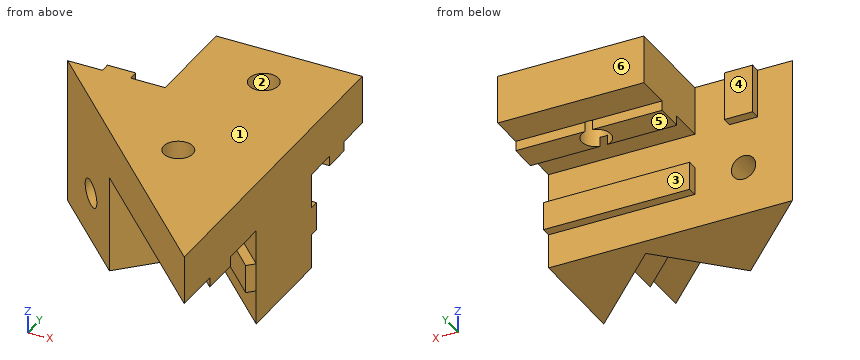
from build123d import *

# Parameters (mm, degrees)
MAIN_DEPTH          = 15
SKETCH4_W           = 15
SKETCH4_H           = 10
CUT_EXTRUDE2_DEPTH  = 10
SKETCH2_W           = 15
SKETCH2_H           = 2.9
BOSS_EXTRUDE3_DEPTH = 1
SKETCH5_W           = 2.9
SKETCH5_H           = 12.715728752
BOSS_EXTRUDE4_DEPTH = 1
SKETCH6_R           = 1.5
BOSS_EXTRUDE5_DEPTH = 5
BOSS_EXTRUDE6_DEPTH = 1
SKETCH8_W           = 2.9
SKETCH8_H           = 10
BOSS_EXTRUDE7_DEPTH = 1
SKETCH9_W           = 1
SKETCH9_H           = 2.9
BOSS_EXTRUDE8_DEPTH = 10
SKETCH11_R          = 1.25
CUT_EXTRUDE4_DEPTH  = 26
SKETCH12_R          = 1.5
CUT_EXTRUDE5_DEPTH  = 16
SKETCH13_W          = 15
SKETCH13_H          = 2.9
BOSS_EXTRUDE9_DEPTH = 1
SKETCH15_W          = 10
SKETCH15_H          = 10
CUT_EXTRUDE7_DEPTH  = 11
SKETCH16_R          = 1.5
CUT_EXTRUDE8_DEPTH  = 16
SKETCH14_W          = 30.791050847
SKETCH14_H          = 42.890305085
CUT_EXTRUDE6_DEPTH  = 26


with BuildPart() as part:
    # Sketch1 → Main (new body)
    with BuildSketch(Plane.XY):
        Polygon((0, 0), (-10, 0), (-10, 10), (-25, 10), (-25, -10.857864376), (-16.008621971, -1.866486348), (-8.937554159, -8.937554159), align=None)
    extrude(amount=MAIN_DEPTH)

    # Sketch4 → Cut-Extrude2 (cut)
    with BuildSketch(Plane(origin=(0, 0, 0), x_dir=(-1, 0, 0), z_dir=(0, 0, -1))):
        with Locations((17.5, 5)):
            Rectangle(SKETCH4_W, SKETCH4_H)
    extrude(amount=-CUT_EXTRUDE2_DEPTH, mode=Mode.SUBTRACT)

    # Sketch2 → Boss-Extrude3 (add)
    with BuildSketch(Plane(origin=(0, 0, 10), x_dir=(-1, 0, 0), z_dir=(0, 0, -1))):
        with Locations((17.5, 5)):
            Rectangle(SKETCH2_W, SKETCH2_H)
    extrude(amount=BOSS_EXTRUDE3_DEPTH)

    # Sketch5 → Boss-Extrude4 (add)
    with BuildSketch(Plane(origin=(-7.071067812, 7.071067812, 0), x_dir=(0, 0, -1), z_dir=(0.707106781, -0.707106781, 0))):
        with Locations((-5, -18.997474683)):
            Rectangle(SKETCH5_W, SKETCH5_H)
    extrude(amount=BOSS_EXTRUDE4_DEPTH)

    # Sketch6 → Boss-Extrude5 (add)
    with BuildSketch(Plane.XY.offset(10)):
        Polygon((-25, -10.857864376), (-16.008621971, -1.866486348), (-8.937554159, -8.937554159), (-25, -25), align=None)
        with Locations((-16.008621971, -8.937554159)):
            Circle(SKETCH6_R, mode=Mode.SUBTRACT)
    extrude(amount=BOSS_EXTRUDE5_DEPTH)

    # Sketch7 → Boss-Extrude6 (add)
    with BuildSketch(Plane(origin=(0, 0, 10), x_dir=(-1, 0, 0), z_dir=(0, 0, -1))):
        Polygon((13.498392898, -4.376715421), (25, -15.878322523), (25, -19.979541854), (11.447783233, -6.427325086), align=None)
    extrude(amount=BOSS_EXTRUDE6_DEPTH)

    # Sketch8 → Boss-Extrude7 (add)
    with BuildSketch(Plane(origin=(0, 0, 0), x_dir=(1, 0, 0), z_dir=(0, 1, 0))):
        with Locations((-5, -10)):
            Rectangle(SKETCH8_W, SKETCH8_H)
    extrude(amount=BOSS_EXTRUDE7_DEPTH)

    # Sketch11 → Cut-Extrude4 (cut, through all)
    with BuildSketch(Plane(origin=(0, 0, 0), x_dir=(1, 0, 0), z_dir=(0, 1, 0))):
        with Locations((-5, -5)):
            Circle(SKETCH11_R)
    extrude(amount=-CUT_EXTRUDE4_DEPTH, mode=Mode.SUBTRACT)

    # Sketch12 → Cut-Extrude5 (cut, through all)
    with BuildSketch(Plane.XY.offset(15)):
        with Locations((-16.008621971, -8.937554159)):
            Circle(SKETCH12_R)
    extrude(amount=-CUT_EXTRUDE5_DEPTH, mode=Mode.SUBTRACT)

    # Sketch13 → Boss-Extrude9 (add)
    with BuildSketch(Plane(origin=(0, 0, 0), x_dir=(1, 0, 0), z_dir=(0, 1, 0))):
        with Locations((-17.5, -5)):
            Rectangle(SKETCH13_W, SKETCH13_H)
    extrude(amount=BOSS_EXTRUDE9_DEPTH)


with BuildPart() as body_2:
    # Sketch9 → Boss-Extrude8 (new body)
    with BuildSketch(Plane.XY.offset(15)):
        with Locations((-9.5, 5)):
            Rectangle(SKETCH9_W, SKETCH9_H)
    extrude(amount=-BOSS_EXTRUDE8_DEPTH)


with BuildPart() as cut_extrude7_tool:
    # Sketch15 → Cut-Extrude7 (new body, through all)
    with BuildSketch(Plane(origin=(0, 0, 10), x_dir=(-1, 0, 0), z_dir=(0, 0, -1))):
        with Locations((5, 5)):
            Rectangle(SKETCH15_W, SKETCH15_H)
    extrude(amount=CUT_EXTRUDE7_DEPTH)


with BuildPart() as part_1:
    add(part.part)

    # Cut-Extrude7: cut by cut_extrude7_tool
    add(cut_extrude7_tool.part, mode=Mode.SUBTRACT)

    # Sketch16 → Cut-Extrude8 (cut, through all)
    with BuildSketch(Plane.XY.offset(15)):
        with Locations((-17.5, 5)):
            Circle(SKETCH16_R)
    extrude(amount=-CUT_EXTRUDE8_DEPTH, mode=Mode.SUBTRACT)


with BuildPart() as body_2_1:
    add(body_2.part)

    # Cut-Extrude7: cut by cut_extrude7_tool
    add(cut_extrude7_tool.part, mode=Mode.SUBTRACT)


with BuildPart() as body_3:
    # Mirror1: mirrored copy
    add(part_1.part.mirror(Plane.ZY.offset(30)))


with BuildPart() as cut_extrude6_tool:
    # Sketch14 → Cut-Extrude6 (new body, through all)
    with BuildSketch(Plane(origin=(-25, 0, -10), x_dir=(0, 0, -1), z_dir=(1, 0, 0))):
        with Locations((-11.471050848, -6.763186441)):
            Rectangle(SKETCH14_W, SKETCH14_H)
    extrude(amount=CUT_EXTRUDE6_DEPTH)


with BuildPart() as part_2:
    add(part_1.part)

    # Cut-Extrude6: cut by cut_extrude6_tool
    add(cut_extrude6_tool.part, mode=Mode.SUBTRACT)


with BuildPart() as body_2_2:
    add(body_2_1.part)

    # Cut-Extrude6: cut by cut_extrude6_tool
    add(cut_extrude6_tool.part, mode=Mode.SUBTRACT)


solid = body_3.part
Could you check a few things on this model? Use its own coordinates, in mm. Face numbers are marked on the shaded views. A direction names the side the tool comes from. Coordinates: 2 decimals unless noted, no trailing zeros. Order: outer loops, then holes, each group sorted by start corner. A loop starts at its lowest first (then second) coordinate and runs counter-clockwise, first axis right, second up. Notation, with made-up numbers: (63.5, -30.5) - (120.5, -30.5) arc R26 cw to (120.5, -9.5) - close; hole circle Ø2 at (53, -16.5). An arc over 180 degrees is marked (long way). Answer in a Markdown table with one row per item. Add a question column.
(1) If we mould it in two halves opening along Y, with no side actions, what happens to the marked faces 1, 2 and 3? For each: released by +Y, released by -Y, zero draft, split by the parting line, or undercut.
(2) If we section it at D-D, the plane z = 11: Please give me the cut outline in (x, y).
(3) Will these pins go through, and if not, where does the flat tip stop? pin 1 (0.8 mm diameter, centred on x = -46, z = 9.5, fed in from -Y); pin 2 (2 mm diameter, centred on x = -49.5, z = 7.5, fed in from -Y); pin 3 (10.5 mm diameter, centred on x = -42, y = -15.5, fed in from -Z); pin 4 (4 mm diameter, centred on x = -44.5, y = 1.5, fed in from -Z).
(4) If we section it at C-C, the plane z = 5: Please give me the cut outline in (x, y).
(5) On a 3-axis mill with a long thin cutter (end or side, diameter ignored), from which of +Z, -Z, +X, -X, +Y, -Y can I reach the whole of each face in a straight line? I mean the marked faces 4, 5 and 6. Say none if no direction works.
(6) I need wall thicknesses on L1, parallel to X at y = 5, z = 13.7; L2, parallel to X at y = -2.75, z = 5; L3, parallel to Z at x = -55, y = -1.25. Which ranges of each line are inside material? Lowest first, please.
(7) If we section it at B-B, the plane x = -54.25: Please give me the cut outline in (y, z), then the cut area to 4 significant figures.
(8) If we section it at A-A, the plane y = 5: Please give me the cut outline in (x, z), then the cut area to 3 significant figures.
Results are:
| question | item | result |
|---|---|---|
| 1 | face 1 | zero draft |
| 1 | face 2 | undercut |
| 1 | face 3 | released by +Y |
| 2 | outline | (-60, 0) - (-35, -25) - (-35, 10) - (-50, 10) - (-50, 0) - (-53.55, 0) - (-53.55, 1) - (-56.45, 1) - (-56.45, 0) - close; hole circle Ø3 at (-43.99, -8.94); hole circle Ø3 at (-42.5, 5) |
| 3 | pin 1 | stops at y = -9.38 |
| 3 | pin 2 | stops at y = -8.38 |
| 3 | pin 3 | stops at z = 9 |
| 3 | pin 4 | stops at z = 0 |
| 4 | outline | (-60, 0) - (-56.25, -3.75) - (-56.25, 0) - close; (-53.75, -6.25) - (-51.06, -8.94) - (-44.7, -2.57) - (-35.71, -11.56) - (-35, -10.86) - (-35, 1) - (-50, 1) - (-50, 0) - (-53.75, 0) - close |
| 5 | face 4 | +Z, -Z, -X, +Y |
| 5 | face 5 | -Z, +X, -X, +Y |
| 5 | face 6 | +Z, -Z, +X, -X, +Y |
| 6 | L1 | x = -50 to -44, -41 to -35 |
| 6 | L2 | x = -57.25 to -56.25, -53.75 to -44.87, -44.52 to -35 |
| 6 | L3 | z = 0 to 3.75, 6.25 to 15 |
| 7 | outline | (-5.75, 0) - (0, 0) - (0, 4) - (-5.75, 4) - close; (-5.75, 6) - (0, 6) - (0, 10) - (1, 10) - (1, 15) - (-5.75, 15) - close |
| 7 | area | 79.75 mm2 |
| 8 | outline | (-50, 9) - (-44, 9) - (-44, 15) - (-50, 15) - close; (-41, 9) - (-35, 9) - (-35, 15) - (-41, 15) - close |
| 8 | area | 72.0 mm2 |
